The model under review builds one solid part; all positions refer to its coordinate system, in mm. Coordinates: 2 decimals unless noted, no trailing zeros. Loops run counter-clockwise (first coordinate to the right, second up) from the corner with the lowest first, then second, coordinate; pieces in that order, holes last. Notation, with made-up numbers: (50, 62) - (82, 62) arc R22 ccw to (82, 85) - close; hole circle Ø2 at (-34.5, 21.25). An arc over 180 degrees is marked (long way). Answer in a Markdown table with one row per item. Add a question column.
(1) We need section A-A on y = 3. Write out the cut boundary in (x, z), plus the area to 3 significant figures.
(2) For line 1 along Y through (x, z) = (17, 69); line 2 along X through (y, z) = (-2, 380); line 3 along Z through (x, y) = (-14.5, -5.5), list the stretches that pass through material, from the lowest coordinate up.
(3) For P1, Ø5, axis at y = -3, z = 189.5, coming from the -X side; P2, Ø3, axis at y = 0.5, z = 300, coming from the -X side; P3, Ø5, axis at x = 18, y = 4, coming from the -Z side, all flat-tipped, find the tip position at first contact; note any pin that passes through.
from build123d import *

# Parameters (mm, degrees)
F1_DEPTH = 6.35
F2_DEPTH = 6.35
F3_SIZE2 = 6.34999
F3_SIZE  = 6.34999


# Not quite as in the source:
# - a fillet or chamfer is up to 0.001 mm smaller than in the source, because OpenCascade refuses the exact size


with BuildPart() as f1:
    # F0 (on Front) → F1 (new body)
    with BuildSketch(Plane.XZ):
        Polygon((-17.139416188, 28.1973872334), (-27.9807504267, 3.4191238228), (0, -37.7674587071), (27.964355424, 3.4191238228), (17.08493568, 28.1973872334), (17.08493568, 469.1244959831), (0, 506.7884922028), (-17.139416188, 469.1244959831), align=None)
    extrude(amount=F1_DEPTH)

    # F2 (add): a face of the model
    f2_faces = [f1.faces().sort_by_distance(p)[0] for p in [
        (-0.0248835797, 0, 225.9211420486),
    ]]
    extrude(f2_faces, amount=F2_DEPTH)

    # F3 (size 6.35 and 6.35 in the source; OpenCascade refuses exactly that, so slightly less here)
    f3_edges = [f1.edges().sort_by_distance(p)[0] for p in [
        (-22.560083, -6.35, 15.808256),
        (-13.990375, -6.35, -17.174167),
        (13.982178, -6.35, -17.174167),
        (22.524646, -6.35, 15.808256),
        (17.084936, -6.35, 248.660942),
        (8.542468, -6.35, 487.956494),
        (-8.569708, -6.35, 487.956494),
        (-17.139416, -6.35, 248.660942),
        (-22.560083, 6.35, 15.808256),
        (-13.990375, 6.35, -17.174167),
        (13.982178, 6.35, -17.174167),
        (22.524646, 6.35, 15.808256),
        (17.084936, 6.35, 248.660942),
        (8.542468, 6.35, 487.956494),
        (-8.569708, 6.35, 487.956494),
        (-17.139416, 6.35, 248.660942),
    ]]
    chamfer(f3_edges, length=F3_SIZE, length2=F3_SIZE2)


solid = f1.part
Outcome:
| question | item | result |
|---|---|---|
| 1 | outline | (-24.57, 3.73) - (0, -32.43) - (24.55, 3.73) - (14.08, 27.57) - (14.08, 468.48) - (0, 499.54) - (-14.14, 468.47) - (-14.14, 27.57) - close |
| 1 | area | 14,700 mm² |
| 2 | line 1 | -0.08 to 0.08 |
| 2 | line 2 | -15.14 to 15.08 |
| 2 | line 3 | -6.64 to 20.51 |
| 3 | P1 | x = -16.64 |
| 3 | P2 | x = -17.14 |
| 3 | P3 | z = -9.91 |
